from build123d import *

# Parameters (mm, degrees)
SKETCH1_W                      = 20
SKETCH1_H                      = 20
BOSS_EXTRUDE1_DEPTH            = 1.5
M2_CLEARANCE_HOLE1_D           = 2.4
M2_CLEARANCE_HOLE1_CSINK_D     = 2.45
M2_CLEARANCE_HOLE1_CSINK_ANGLE = 90
FILLET1_R                      = 1
CUT_EXTRUDE1_REACH             = 16.221
SKETCH2_R                      = 4.1
SKETCH6_R                      = 5.45
SKETCH6_R_2                    = 4.1
BOSS_EXTRUDE2_DEPTH            = 2.3
CHAMFER1_SIZE                  = 0.5


with BuildPart() as part:
    # Sketch1 → Boss-Extrude1 (new body)
    with BuildSketch(Plane(origin=(0, 0, 0), x_dir=(1, 0, 0), z_dir=(0, 1, 0))):
        Rectangle(SKETCH1_W, SKETCH1_H)
    extrude(amount=BOSS_EXTRUDE1_DEPTH)

    # M2 Clearance Hole1 (through all)
    with Locations(Plane(origin=(0, 1.5, 0), x_dir=(1, 0, 0), z_dir=(0, 1, 0))):
        with Locations((-6, 6), (6, 6), (-6, -6), (6, -6)):
            CounterSinkHole(M2_CLEARANCE_HOLE1_D / 2, M2_CLEARANCE_HOLE1_CSINK_D / 2, counter_sink_angle=M2_CLEARANCE_HOLE1_CSINK_ANGLE)

    # Fillet1
    fillet1_edges = [part.edges().sort_by_distance(p)[0] for p in [
        (-10, 1.5, 0),
        (0, 1.5, 10),
        (10, 1.5, 0),
        (0, 1.5, -10),
    ]]
    fillet(fillet1_edges, radius=FILLET1_R)

    # Sketch2 → Cut-Extrude1 (cut, up to next)
    with BuildSketch(Plane(origin=(0, 1.5, 0), x_dir=(1, 0, 0), z_dir=(0, 1, 0)), mode=Mode.PRIVATE) as cut_extrude1_sk1:
        with Locations(Location((0, 0, 0), (0, 0, 270))):
            Circle(SKETCH2_R)
    cut_extrude1_tool1 = extrude(cut_extrude1_sk1.sketch, amount=-CUT_EXTRUDE1_REACH, mode=Mode.PRIVATE) & part.part
    add(cut_extrude1_tool1.solids().sort_by_distance((0, 1.5, 0))[0], mode=Mode.SUBTRACT)

    # Sketch6 → Boss-Extrude2 (add)
    with BuildSketch(Plane.XZ):
        with Locations(Location((0, 0, 0), (0, 0, 270))):
            Circle(SKETCH6_R)
        with Locations(Location((0, 0, 0), (0, 0, 90))):
            Circle(SKETCH6_R_2, mode=Mode.SUBTRACT)
    extrude(amount=BOSS_EXTRUDE2_DEPTH)

    # Chamfer1
    chamfer1_edges = [part.edges().sort_by_distance(p)[0] for p in [
        (0, -2.3, 5.45),
    ]]
    chamfer(chamfer1_edges, length=CHAMFER1_SIZE)


solid = part.part
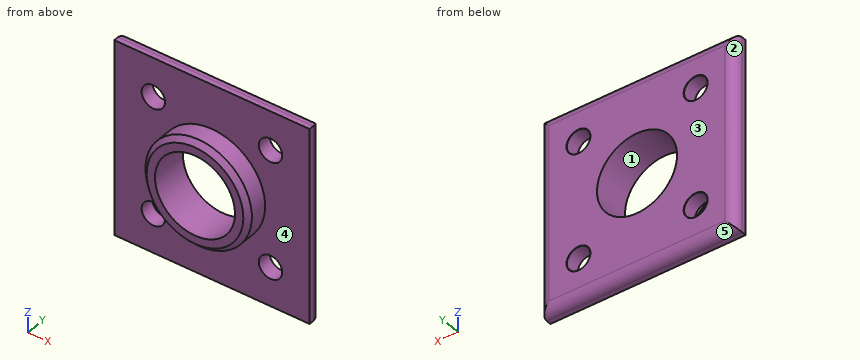
Geometry check sheet. Reference: the model listing, model coordinates, mm. Face numbers are marked on the shaded views. A direction names the side the tool comes from. Give positions to 0.01 mm unless a question says otherwise; leave off trailing zeros. Order: outer loops, then holes, each group sorted by start corner. A loop starts at its lowest first (then second) coordinate and runs counter-clockwise, first axis right, second up.
1. Draft check along X on the marked faces 1, 2 and 3. Enter one of: pulls with the +X half, pulls with the -X half, needs draft (parallel to the pull), parting line crosses it, or undercut.
Completed:
face 1: undercut
face 2: pulls with the -X half
face 3: needs draft
2. Access from +Z, -Z, +X, -X, +Y, -Y to the whole of each face (thin tool, end or side, straight path). Record for the marked faces 4 and 5.
Completed:
face 4: -Y
face 5: -Z, +X, -X, +Y
3. Sectioned sample at D-D (x = -6). Record the boundary of the cut face in (y, z) (3 decimals), then the cut area to 3 significant figures.
Completed:
outline: (0, -10) - (0.5, -10) arc R1 ccw to (1.5, -9) - (1.5, -7.225) - (1.475, -7.2) - (0, -7.2) - close; (0, -4.8) - (1.475, -4.8) - (1.5, -4.775) - (1.5, 4.775) - (1.475, 4.8) - (0, 4.8) - close; (0, 7.2) - (1.475, 7.2) - (1.5, 7.225) - (1.5, 9) arc R1 ccw to (0.5, 10) - (0, 10) - close
area: 22.4 mm2
4. Scan lines: line 1 (X direction, y = 0.3, z = -6); line 2 (X direction, y = 0.9, z = 6). Record each from-to range of solid material in increasing order.
Completed:
line 1: x = -10 to -7.2, -4.8 to 4.8, 7.2 to 10
line 2: x = -9.92 to -7.2, -4.8 to 4.8, 7.2 to 9.92
5. Sectioned sample at B-B (x = 0). Record the boundary of the cut face in (y, z).
Completed:
outline: (-2.3, -4.95) - (-1.8, -5.45) - (0, -5.45) - (0, -10) - (0.5, -10) arc R1 ccw to (1.5, -9) - (1.5, -4.1) - (-2.3, -4.1) - close; (-2.3, 4.1) - (1.5, 4.1) - (1.5, 9) arc R1 ccw to (0.5, 10) - (0, 10) - (0, 5.45) - (-1.8, 5.45) - (-2.3, 4.95) - close
6. Sectioned sample at A-A (z = 6). Record the boundary of the cut face in (x, y) (3 decimals), then the cut area to 3 significant figures.
Completed:
outline: (-10, 0) - (-7.2, 0) - (-7.2, 1.475) - (-7.225, 1.5) - (-9, 1.5) arc R1 ccw to (-10, 0.5) - close; (-4.8, 0) - (4.8, 0) - (4.8, 1.475) - (4.775, 1.5) - (-4.775, 1.5) - (-4.8, 1.475) - close; (7.2, 0) - (10, 0) - (10, 0.5) arc R1 ccw to (9, 1.5) - (7.225, 1.5) - (7.2, 1.475) - close
area: 22.4 mm2
7. Sectioned sample at C-C (z = 0). Record the boundary of the cut face in (x, y).
Completed:
outline: (-10, 0) - (-5.45, 0) - (-5.45, -1.8) - (-4.95, -2.3) - (-4.1, -2.3) - (-4.1, 1.5) - (-9, 1.5) arc R1 ccw to (-10, 0.5) - close; (4.1, -2.3) - (4.95, -2.3) - (5.45, -1.8) - (5.45, 0) - (10, 0) - (10, 0.5) arc R1 ccw to (9, 1.5) - (4.1, 1.5) - close
8. Depth check by flat-ended pin: pin 1 (4 mm diameter, centred on x = -6, z = 6, fed in from +Y); pin 2 (3 mm diameter, centred on x = -6, z = -6, fed in from -Y); pin 3 (1.5 mm diameter, centred on y = -1, z = 2, fed in from -X); pin 4 (1.5 mm diameter, centred on y = -1, z = 2, fed in from +X). Enter the tip coordinate at first touch or a pass-through.
Completed:
pin 1: stops at y = 1.5
pin 2: stops at y = 0
pin 3: stops at x = -5.3
pin 4: stops at x = 5.3
